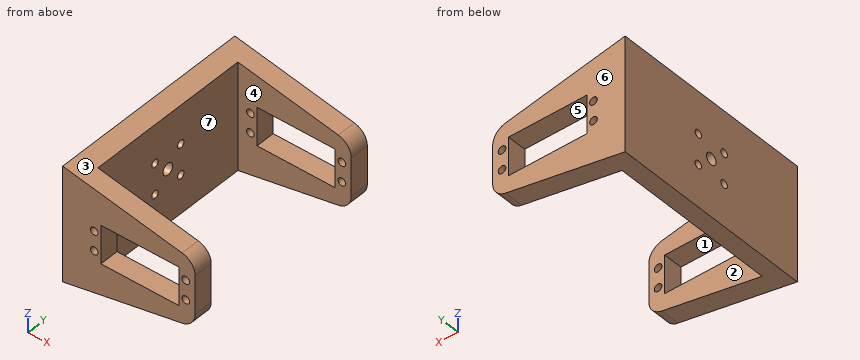
Autodesk Inventor part; units mm, degrees
ref_plane "Work Plane1" through (0, -43.44, 0) normal (0, -1, 0) x (1, 0, 0)
ref_plane "YZ Plane" through (0, 0, 0) normal (1, 0, 0) x (0, 1, 0)
ref_plane "XZ Plane" through (0, 0, 0) normal (0, 1, 0) x (-1, 0, 0)
sketch "Sketch1" plane through (0, 0, 0) normal (0, 1, 0) x (-1, 0, 0)
  line L0 (20.45, 10) -> (-20.45, 10)
  line L1 (-20.45, 10) -> (-20.45, -10)
  line L2 (-20.45, -10) -> (20.45, -10)
  line L3 (20.45, -10) -> (20.45, 10)
  line L4 (20.45, 10) -> (-20.45, -10) construction
  line L5 (-20.45, 10) -> (20.45, -10) construction
  line L6 (-20.45, 10) -> (-23.9, 10)
  line L7 (-23.9, 10) -> (-23.9, 5.1) construction
  circle A0 centre (-23.9, 5.1) radius 2
  line L8 (-23.9, 5.1) -> (-20.45, 5.1) construction
  line L9 (0, 0) -> (-20.45, 0) construction
  line L10 (-20.45, -10) -> (-23.9, -10)
  line L11 (-23.9, -10) -> (-23.9, -5.1) construction
  circle A1 centre (-23.9, -5.1) radius 2
  line L12 (-23.9, -5.1) -> (-20.45, -5.1) construction
  arc A2 (-28.8, -10) -> (-21.9997, -18.2049) centre (-20.45, -10) ccw
  line L13 (-28.8, 0) -> (-28.8, -10)
  line L14 (0, 0) -> (0, -10) construction
  circle A3 centre (23.9, 5.1) radius 2
  line L15 (23.9, 5.1) -> (20.45, 5.1) construction
  circle A4 centre (23.9, -5.1) radius 2
  line L16 (23.9, -5.1) -> (20.45, -5.1) construction
  line L17 (40.45, -30) -> (-21.9997, -18.2049)
  line L18 (0, 0) -> (-20.45, 0) construction
  line L19 (30.45, 0) -> (30.45, -28.1113)
  line L20 (40.45, -28.1113) -> (40.45, 0)
  line L21 (40.45, 0) -> (40.45, -30)
  arc A5 (-21.9997, 18.2049) -> (-28.8, 10) centre (-20.45, 10) ccw
  line L22 (40.45, 30) -> (-21.9997, 18.2049)
  line L23 (30.45, 0) -> (30.45, 28.1113)
  line L24 (40.45, 28.1113) -> (40.45, 0)
  line L25 (40.45, 0) -> (40.45, 30)
  line L26 (-28.8, 10) -> (-28.8, 0)
  point P0 (20.45, 0)
  dimension "d0" = 40.9
  dimension "d1" = 20
  dimension "d2" = 3.45
  dimension "d3" = 4.9
  dimension "d4" = 4
  dimension "d10" = 10
extrude "Extrusion1" add sketch "Sketch1" along normal blind 10
ref_plane "Work Plane1" through (0, -43.44, 0) normal (0, -1, 0) x (1, 0, 0)
mirror "Mirror1" about plane through (0, -43.44, 0) normal (0, -1, 0) of "Extrusion1"
extrude "Extrusion2" add sketch "Sketch1" against normal blind 86.88 contours L19 L23 L22 L25 L24 L20 L21 L17
sketch "Sketch2" plane through (-30.45, -86.88, 28.1113) normal (1, 0, 0) x (0, 0, -1)
  line L0 (56.2225, 86.88) -> (56.2225, 0)
  line L1 (0, 0) -> (56.2225, 0)
  line L2 (56.2225, 0) -> (56.2225, 86.88)
  line L3 (56.2225, 86.88) -> (0, 86.88)
  line L4 (0, 86.88) -> (0, 0)
  line L5 (0, 86.88) -> (0, 0) construction
  line L6 (0, 0) -> (56.2225, 86.88) construction
  circle A0 centre (28.1113, 43.44) radius 3
  line L7 (20.1113, 35.44) -> (36.1113, 35.44) construction
  line L8 (36.1113, 35.44) -> (36.1113, 51.44) construction
  line L9 (36.1113, 51.44) -> (20.1113, 51.44) construction
  line L10 (20.1113, 51.44) -> (20.1113, 35.44) construction
  line L11 (20.1113, 35.44) -> (36.1113, 51.44) construction
  line L12 (36.1113, 35.44) -> (20.1113, 51.44) construction
  circle A1 centre (20.1113, 51.44) radius 2
  circle A2 centre (20.1113, 35.44) radius 2
  circle A3 centre (36.1113, 35.44) radius 2
  circle A4 centre (36.1113, 51.44) radius 2
  point P0 (28.1113, 86.88)
  dimension "d13" = 6
  dimension "d24" = 16
  dimension "d25" = 4
extrude "Extrusion3" cut sketch "Sketch2" against normal blind 10 contours A0 | A1 | A2 | A3 | A4
properties part number "Hand-End Fork" material "Acrylic, Clear"
Can you work these out from the model? Positions are in its coordinate system, mm. Face numbers are marked on the shaded views. A direction names the side the tool comes from. Round coordinates to 2 decimals unless told otherwise and drop trailing zeros. Write each loop counter-clockwise with the first axis right and the second up, starting at its lowest first coordinate (ties: lowest second). Pieces come first, ordered by that corner, then holes. Notation, with made-up numbers: (42.25, 63) - (71.25, 63) arc R24 cw to (71.25, 95) - close; hole circle Ø3 at (-20.75, -4). An arc over 180 degrees is marked (long way). Write each question's results on one line, items separated by ' | '. Start each with the question number.
1) Suppose I cut it at C-C (x = -23.9). List the corners of the cut face in (y, z) for me.
2) Suppose I cut it at D-D (x = 4). List the corners of the cut face in (y, z) for me, and give its area (3 significant figures).
3) Which directions (+Z, -Z, +X, -X, +Y, -Y) give clear straight access to the entire face, cutting with the end or side of a thin tool? Please do the marked faces 1, 2 and 3.
4) For pin 1 Ø1.5 at (y, z) = (-57, -12.5) entering from +X; pin 2 Ø3 at (x, z) = (23.9, -5.1) entering from +Y; pin 3 Ø11 at (x, y) = (0, 5) entering from +Z; pin 4 Ø8 at (x, y) = (2, 4.5) entering from -Z, each with a flat end and sliding along its axis, tell me the tip position at first contact or that it passes through.
5) We'd pull the mould along Y, two halves only. Please class the marked faces 4, 5, 6 and 7: released by +Y, released by -Y, zero draft, split by the parting line, or undercut.
6) Suppose I cut it at B-B (y = 2.5). List the corners of the cut face in (x, z) for me.
7) Suppose I cut it at A-A (z = 0). List the corners of the cut face in (x, y) for me, and give its area (3 significant figures).
8) Please list where these lines run through material, in increasing order: line 1 (X direction, y = -92, z = -5); line 2 (Y direction, x = -35, z = 0); line 3 (Y direction, x = -0.5, z = 22).
Here are the results:
1) outline: (-96.88, -26.87) - (-86.88, -26.87) - (-86.88, -7.1) - (-96.88, -7.1) - close; (-96.88, -3.1) - (-86.88, -3.1) - (-86.88, 3.1) - (-96.88, 3.1) - close; (-96.88, 7.1) - (-86.88, 7.1) - (-86.88, 26.87) - (-96.88, 26.87) - close; (0, -26.87) - (10, -26.87) - (10, -7.1) - (0, -7.1) - close; (0, -3.1) - (10, -3.1) - (10, 3.1) - (0, 3.1) - close; (0, 7.1) - (10, 7.1) - (10, 26.87) - (0, 26.87) - close
2) outline: (-96.88, -21.6) - (-86.88, -21.6) - (-86.88, -10) - (-96.88, -10) - close; (-96.88, 10) - (-86.88, 10) - (-86.88, 21.6) - (-96.88, 21.6) - close; (0, -21.6) - (10, -21.6) - (10, -10) - (0, -10) - close; (0, 10) - (10, 10) - (10, 21.6) - (0, 21.6) - close | area: 464 mm2
3) face 1: +Y, -Y | face 2: +Z, -Z, +X | face 3: +Z, +X, +Y, -Y
4) pin 1: stops at x = -30.45 | pin 2: passes through | pin 3: stops at z = 23.4 | pin 4: stops at z = -22.74
5) face 4: undercut | face 5: zero draft | face 6: released by +Y | face 7: undercut
6) outline: (-40.45, -30) - (22, -18.2) arc R8.35 ccw to (28.8, -10) - (28.8, 10) arc R8.35 ccw to (22, 18.2) - (-40.45, 30) - close; hole circle Ø4 at (-23.9, -5.1); hole circle Ø4 at (-23.9, 5.1); hole (-20.45, -10) - (20.45, -10) - (20.45, 10) - (-20.45, 10) - close; hole circle Ø4 at (23.9, -5.1); hole circle Ø4 at (23.9, 5.1)
7) outline: (-40.45, -96.88) - (-20.45, -96.88) - (-20.45, -86.88) - (-30.45, -86.88) - (-30.45, -46.44) - (-40.45, -46.44) - close; (-40.45, -40.44) - (-30.45, -40.44) - (-30.45, 0) - (-20.45, 0) - (-20.45, 10) - (-40.45, 10) - close; (20.45, -96.88) - (28.8, -96.88) - (28.8, -86.88) - (20.45, -86.88) - close; (20.45, 0) - (28.8, 0) - (28.8, 10) - (20.45, 10) - close | area: 1,380 mm2
8) line 1: x = -40.45 to -25.9, -21.9 to -20.45, 20.45 to 21.9, 25.9 to 28.8 | line 2: y = -96.88 to -46.44, -40.44 to 10 | line 3: y = -96.88 to -86.88, 0 to 10
